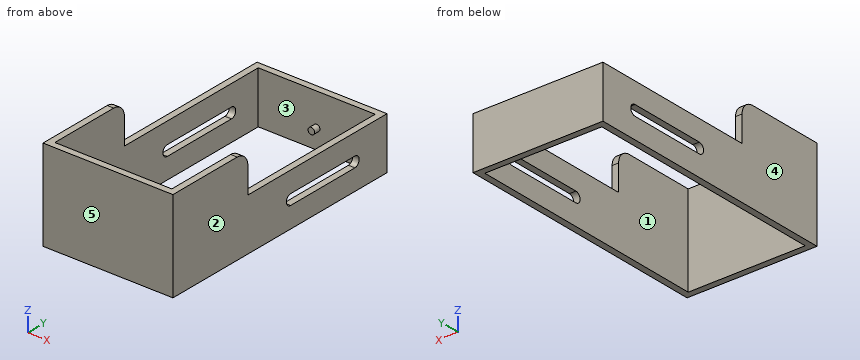
```python
from build123d import *

# Parameters (mm, degrees)
SKETCH1_W               = 100
SKETCH1_H               = 200
SKETCH1_W_2             = 90
SKETCH1_H_2             = 190
BOSS_EXTRUDE1_DEPTH     = 70
SKETCH2_W               = 30
SKETCH2_H               = 130
CUT_EXTRUDE1_DEPTH      = 1
CUT_EXTRUDE1_DEPTH_BACK = 101
FILLET1_R               = 10
SKETCH3_R               = 2.5
BOSS_EXTRUDE2_DEPTH     = 5
CUT_EXTRUDE2_DEPTH      = 1
CUT_EXTRUDE2_DEPTH_BACK = 101


with BuildPart() as part:
    # Sketch1 → Boss-Extrude1 (new body)
    with BuildSketch(Plane.XY):
        Rectangle(SKETCH1_W, SKETCH1_H)
        Rectangle(SKETCH1_W_2, SKETCH1_H_2, mode=Mode.SUBTRACT)
    extrude(amount=BOSS_EXTRUDE1_DEPTH)

    # Sketch2 → Cut-Extrude1 (cut, two sides)
    with BuildSketch(Plane(origin=(50, 0, 0), x_dir=(0, 0, -1), z_dir=(1, 0, 0))) as cut_extrude1_sk:
        with Locations((-55, 35)):
            Rectangle(SKETCH2_W, SKETCH2_H)
    extrude(amount=CUT_EXTRUDE1_DEPTH, mode=Mode.SUBTRACT)
    extrude(cut_extrude1_sk.sketch, amount=-CUT_EXTRUDE1_DEPTH_BACK, mode=Mode.SUBTRACT)

    # Fillet1
    fillet1_edges = [part.edges().sort_by_distance(p)[0] for p in [
        (47.5, -30, 70),
        (-47.5, -30, 70),
    ]]
    fillet(fillet1_edges, radius=FILLET1_R)

    # Sketch3 → Boss-Extrude2 (add)
    with BuildSketch(Plane.XZ.offset(-95)):
        with Locations((0, 15)):
            Circle(SKETCH3_R)
    extrude(amount=BOSS_EXTRUDE2_DEPTH)

    # Sketch4 → Cut-Extrude2 (cut, two sides)
    with BuildSketch(Plane.ZY.offset(50)) as cut_extrude2_sk:
        with BuildLine():
            Line((16, 10), (16, 70))
            ThreePointArc((16, 70), (20, 74), (24, 70))
            Line((24, 70), (24, 10))
            ThreePointArc((24, 10), (20, 6), (16, 10))
        make_face()
    extrude(amount=CUT_EXTRUDE2_DEPTH, mode=Mode.SUBTRACT)
    extrude(cut_extrude2_sk.sketch, amount=-CUT_EXTRUDE2_DEPTH_BACK, mode=Mode.SUBTRACT)


solid = part.part
```
Design review of the part built by this model. Coordinates are the model's own, in mm. Face numbers are marked on the shaded views. A direction names the side the tool comes from. Give positions to 0.01 mm unless a question says otherwise; leave off trailing zeros. Write each loop counter-clockwise with the first axis right and the second up, starting at its lowest first coordinate (ties: lowest second). Pieces come first, ordered by that corner, then holes. Notation, with made-up numbers: (20.25, 10) -> (27.25, 10) arc R35 cw to (27.25, 46) -> close; hole circle Ø7 at (-8.5, -4). An arc over 180 degrees is marked (long way). Answer in a Markdown table with one row per item.
(1) Mouldability with a two-part tool opening along X and no side actions: class the marked faces 3, 4 and 5 as +X half, -X half, draft (parallel to the pull), parting line (faces both ways), or undercut.
Results:
| item | result |
|---|---|
| face 3 | undercut |
| face 4 | -X half |
| face 5 | draft |
(2) Consider section C-C (x = -20). State the section outline as (y, z) points.
Results:
| item | result |
|---|---|
| outline | (-100, 0) -> (-95, 0) -> (-95, 70) -> (-100, 70) -> close; (95, 0) -> (100, 0) -> (100, 40) -> (95, 40) -> close |
(3) To check wall thickness, follow probe 1 along Y at (x, z) = (-34.5, 25.5); probe 2 along X at (y, z) = (-70.5, 31.5); probe 3 along Y at (x, z) = (-38.5, 65). State the ranges of each line that lie inside material, in increasing order.
Results:
| item | result |
|---|---|
| probe 1 | -100 to -95, 95 to 100 |
| probe 2 | -50 to -45, 45 to 50 |
| probe 3 | -100 to -95 |
(4) Consider section B-B (y = -79). State the section outline as (x, z) points.
Results:
| item | result |
|---|---|
| outline | (-50, 0) -> (-45, 0) -> (-45, 70) -> (-50, 70) -> close; (45, 0) -> (50, 0) -> (50, 70) -> (45, 70) -> close |
(5) Consider section A-A (z = 20). State the section outline as (x, y) points, then the cut area to 3 significant figures.
Results:
| item | result |
|---|---|
| outline | (-50, -100) -> (50, -100) -> (50, 6) -> (45, 6) -> (45, -95) -> (-45, -95) -> (-45, 6) -> (-50, 6) -> close; (-50, 74) -> (-45, 74) -> (-45, 95) -> (45, 95) -> (45, 74) -> (50, 74) -> (50, 100) -> (-50, 100) -> close |
| area | 2,220 mm2 |
(6) For the marked faces 1 and 2, list the 3-axis set-ups (+Z, -Z, +X, -X, +Y, -Y) from which the entire face can be reached by the end or side of a thin tool; tool diameter is ignored.
Results:
| item | result |
|---|---|
| face 1 | +Z, -Z |
| face 2 | +Z, -Z, +X, +Y, -Y |
(7) Clearance check with flat-ended pins moving along their axes: pin 1 (4 mm diameter, centred on x = -48.5, z = 49, fed in from +Y); pin 2 (2.5 mm diameter, centred on x = 46.5, y = 54.5, fed in from +Z). State where each tip first meets the part, or that it passes through.
Results:
| item | result |
|---|---|
| pin 1 | y = -30 |
| pin 2 | z = 40 |
(8) Consider section D-D (y = 67.5). State the section outline as (x, z) points, then the cut area to 3 significant figures.
Results:
| item | result |
|---|---|
| outline | (-50, 0) -> (-45, 0) -> (-45, 16) -> (-50, 16) -> close; (-50, 24) -> (-45, 24) -> (-45, 40) -> (-50, 40) -> close; (45, 0) -> (50, 0) -> (50, 16) -> (45, 16) -> close; (45, 24) -> (50, 24) -> (50, 40) -> (45, 40) -> close |
| area | 320 mm2 |
